Job drawing, mm, ordinate dimensions from the low corner. One solid piece. Give positions to 0.01 mm unless a question says otherwise; leave off trailing zeros. Order: outer loops, then holes, each group sorted by start corner. A loop starts at its lowest first (then second) coordinate and runs counter-clockwise, first axis right, second up. Notation, with made-up numbers: (-16, 11) -> (19, 11) arc R13 cw to (19, 29) -> close; hole circle Ø10 at (20.25, -20.75). An arc over 180 degrees is marked (long way). Write item = value, one per line. Start each with the question number.
(1) Saw through at B-B, the plane z = 2. List the corners of the cut face in (x, y), then the cut area to 3 significant figures.
(2) Probe line 1 along Y through (x, z) = (12, 5); line 2 along Y through (x, z) = (40, 3.75). List the from-to ranges inside material, lowest first. Write a range as from..to.
(3) Flat gauge pins, fed straight in: pin 1 (3 mm diameter, centred on x = 84, z = 4.5, fed in from +Y); pin 2 (1 mm diameter, centred on x = 74, z = 7.5, fed in from +Y). Where does each tip first touch, or does it go through?
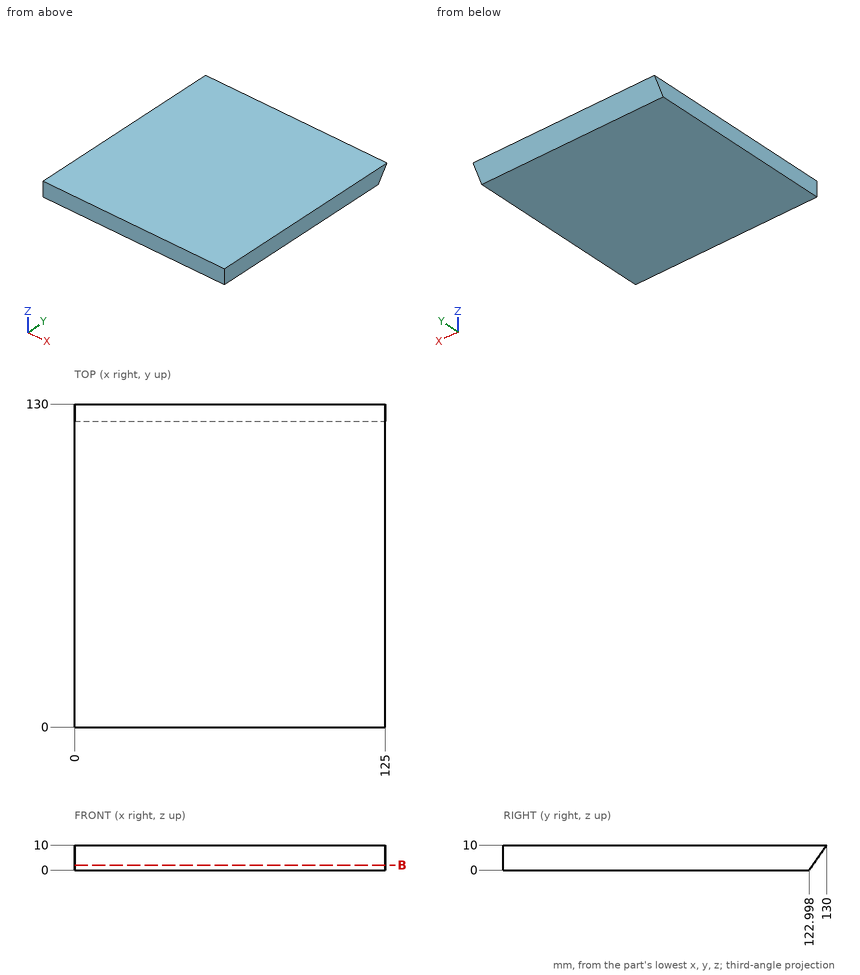
Results list:
q1.outline = (0, 0) -> (125, 0) -> (125, 124.4) -> (0, 124.4) -> close
q1.area = 15,500 mm^2
q2.line_1 = 0..126.5
q2.line_2 = 0..125.62
q3.pin_1 = 127.2
q3.pin_2 = 128.6
